Source: three-view drawing plus pictorial views. Frame: mm from the lowest corner of the part. A direction names the side the tool comes from. Give positions to 0.01 mm unless a question says otherwise; leave off trailing zeros. Loops run counter-clockwise (first coordinate to the right, second up) from the corner with the lowest first, then second, coordinate; pieces in that order, holes last.
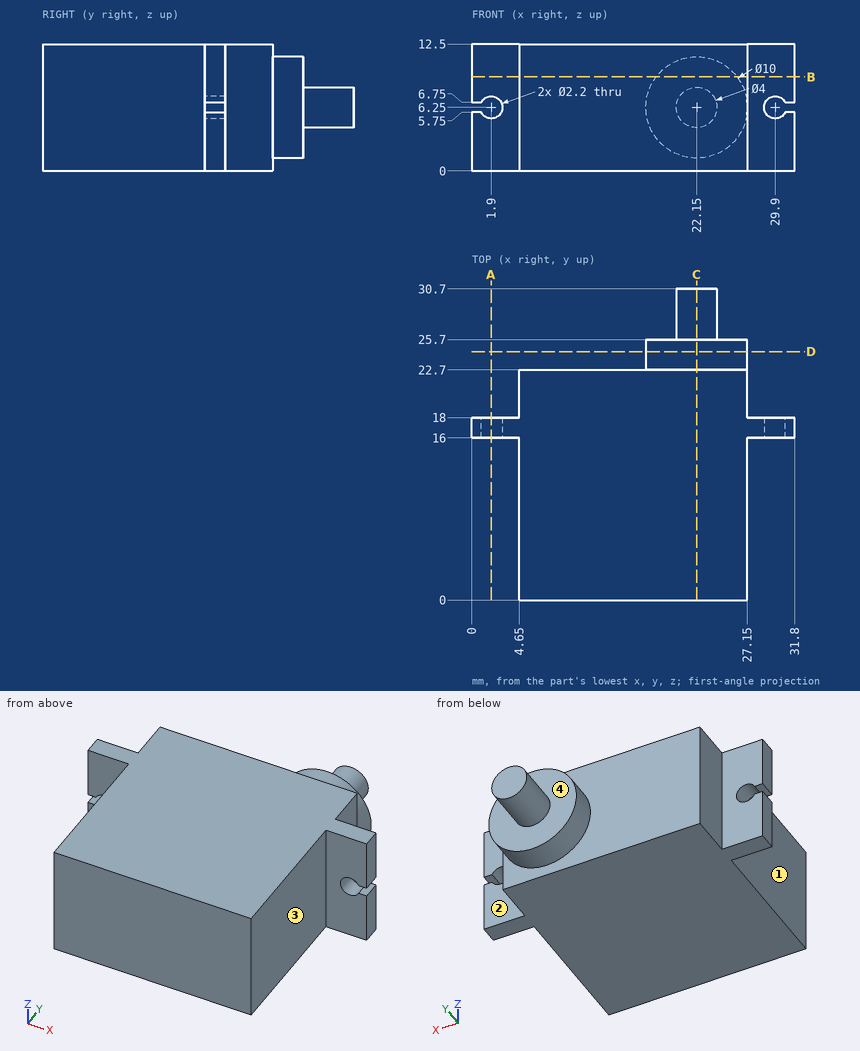
(1) Cut plane C-C (x = 22.15). Return the cut outline in (y, z), and give its area (3 significant figures).
Values follow:
outline: (0, 0) - (22.7, 0) - (22.7, 1.25) - (25.7, 1.25) - (25.7, 4.25) - (30.7, 4.25) - (30.7, 8.25) - (25.7, 8.25) - (25.7, 11.25) - (22.7, 11.25) - (22.7, 12.5) - (0, 12.5) - close
area: 334 mm2
(2) Ray query, probe 1 along Z at (x, y) = (29.9, 17); probe 2 along Y at (x, z) = (25, 7.25); probe 3 along Y at (x, z) = (19, 11.25). Return the intervals inside material, ascending.
Values follow:
probe 1: z = 0 to 5.15, 7.35 to 12.5
probe 2: y = 0 to 25.7
probe 3: y = 0 to 22.7
(3) Cut plane A-A (x = 1.9). Return the cut outline in (y, z).
Values follow:
outline: (16, 0) - (18, 0) - (18, 5.15) - (16, 5.15) - close; (16, 7.35) - (18, 7.35) - (18, 12.5) - (16, 12.5) - close
(4) Pin query (flat end, axial travel): pin 1 Ø2.5 at (x, z) = (1.5, 8) entering from +Y; pin 2 Ø5 at (x, z) = (29.5, 4.5) entering from +Y; pin 3 Ø6 at (y, z) = (25, 4) entering from -X. Return the tip coordinate at first contact, or that it passes through.
Values follow:
pin 1: stops at y = 18
pin 2: stops at y = 22.7
pin 3: stops at x = 4.65
(5) Reachability of the marked faces 1, 2, 3 and 4 from +Z, -Z, +X, -X, +Y, -Y: full face, straight path, thin tool, end or side. Return the list, or none.
Values follow:
face 1: +Z, -Z, -X, -Y
face 2: +Z, -Z, +X, +Y
face 3: +Z, -Z, +X, -Y
face 4: +Y
(6) Cut plane B-B (z = 9.25). Return the cut outline in (x, y).
Values follow:
outline: (0, 16) - (4.65, 16) - (4.65, 0) - (27.15, 0) - (27.15, 16) - (31.8, 16) - (31.8, 18) - (27.15, 18) - (27.15, 22.7) - (26.15, 22.7) - (26.15, 25.7) - (18.15, 25.7) - (18.15, 22.7) - (4.65, 22.7) - (4.65, 18) - (0, 18) - close
(7) Cut plane D-D (y = 24.5). Return the cut outline in (x, z), and give its area (3 significant figures).
Values follow:
outline: circle Ø10 at (22.15, 6.25)
area: 78.5 mm2
